Read the model definition and answer for the solid it produces. Units are mm, in the model's axes. Give positions to 0.01 mm unless a question says otherwise; leave off trailing zeros. Loops run counter-clockwise (first coordinate to the right, second up) from the corner with the lowest first, then second, coordinate; pieces in that order, holes last. Notation, with made-up numbers: (17, 61.25) -> (51, 61.25) arc R19 cw to (51, 69.25) -> close; hole circle Ø4 at (-24, 55). An arc over 180 degrees is marked (long way). One line per item, written item: value. Start each with the question number.
from build123d import *

# Parameters (mm, degrees)
SKETCH1_W      = 9.144
SKETCH1_H      = 4.572
EXTRUDE1_DEPTH = 3.048
SKETCH2_W      = 0.762
SKETCH2_H      = 0.762
EXTRUDE2_DEPTH = 7.62


with BuildPart() as part:
    # Sketch1 → Extrude1 (new body)
    with BuildSketch(Plane(origin=(0, 0, 0), x_dir=(1, 0, 0), z_dir=(0, 1, 0))):
        with Locations((4.572, 2.286)):
            Rectangle(SKETCH1_W, SKETCH1_H)
    extrude(amount=EXTRUDE1_DEPTH)

    # Sketch2 → Extrude2 (add)
    with BuildSketch(Plane(origin=(0, 3.048, 0), x_dir=(1, 0, 0), z_dir=(0, 1, 0))):
        with Locations((3.429, 3.429)):
            Rectangle(SKETCH2_W, SKETCH2_H)
        with Locations((1.143, 3.429)):
            Rectangle(SKETCH2_W, SKETCH2_H)
        with Locations((5.715, 3.429)):
            Rectangle(SKETCH2_W, SKETCH2_H)
        with Locations((8.001, 3.429)):
            Rectangle(SKETCH2_W, SKETCH2_H)
        with Locations((1.143, 1.143)):
            Rectangle(SKETCH2_W, SKETCH2_H)
        with Locations((3.429, 1.143)):
            Rectangle(SKETCH2_W, SKETCH2_H)
        with Locations((5.715, 1.143)):
            Rectangle(SKETCH2_W, SKETCH2_H)
        with Locations((8.001, 1.143)):
            Rectangle(SKETCH2_W, SKETCH2_H)
    extrude(amount=EXTRUDE2_DEPTH)


solid = part.part
Item 1: Section C-C, the plane x = 8.25 is taken. Determine the outline of the cut face in (y, z).
Item 2: Section A-A, the plane y = 5 is taken. State how many separate pieces and enclosed holes the cut face has, plus the area to 3 significant figures.
Item 3: Consider L1, parallel to X at y = 9.25, z = -3.4; L2, parallel to Z at x = 1.25, y = 5.5; L3, parallel to Y at x = 2, z = -3.15. Determine where each line is inside the solid, lowest interval first. Write a range as [from, to].
Item 4: Flat-ended cylindrical pins translate along their axes: pin 1 (0.8 mm diameter, centred on y = 7, z = -3.5, fed in from -X); pin 2 (0.6 mm diameter, centred on y = 7, z = -1, fed in from +X); pin 3 (1 mm diameter, centred on x = 8, y = 8, fed in from -Z). Find the tip coordinate at first contact, or state that the pin passes through.
Item 5: Determine the mould class of faces 1 (the flat face through (0, 2, -2)), 2 (the flat face through (9.144, 2, -2)), 3 (the flat face through (5, 3.048, -2)), 4 (the flat face through (5, 2, 0)) for opening direction X: pulls with the +X half, pulls with the -X half, needs draft (parallel to the pull), parting line crosses it, or undercut.
Item 6: Section D-D, the plane x = 6.5 is taken. Determine the outline of the cut face in (y, z), plus the area to 3 significant figures.
Item 7: Section B-B, the plane z = -1 is taken. Determine the outline of the cut face in (x, y), plus the area to 3 significant figures.
Computed values:
1. outline: (0, -4.57) -> (3.05, -4.57) -> (3.05, -3.81) -> (10.67, -3.81) -> (10.67, -3.05) -> (3.05, -3.05) -> (3.05, -1.52) -> (10.67, -1.52) -> (10.67, -0.76) -> (3.05, -0.76) -> (3.05, 0) -> (0, 0) -> close
2. separate pieces: 8
2. enclosed holes: 0
2. area: 4.65 mm²
3. L1: [0.76, 1.52], [3.05, 3.81], [5.33, 6.1], [7.62, 8.38]
3. L2: [-3.81, -3.05], [-1.52, -0.76]
3. L3: [0, 3.05]
4. pin 1: x = 0.76
4. pin 2: x = 8.38
4. pin 3: z = -3.81
5. face 1: pulls with the -X half
5. face 2: pulls with the +X half
5. face 3: undercut
5. face 4: needs draft
6. outline: (0, -4.57) -> (3.05, -4.57) -> (3.05, 0) -> (0, 0) -> close
6. area: 13.9 mm²
7. outline: (0, 0) -> (9.14, 0) -> (9.14, 3.05) -> (8.38, 3.05) -> (8.38, 10.67) -> (7.62, 10.67) -> (7.62, 3.05) -> (6.1, 3.05) -> (6.1, 10.67) -> (5.33, 10.67) -> (5.33, 3.05) -> (3.81, 3.05) -> (3.81, 10.67) -> (3.05, 10.67) -> (3.05, 3.05) -> (1.52, 3.05) -> (1.52, 10.67) -> (0.76, 10.67) -> (0.76, 3.05) -> (0, 3.05) -> close
7. area: 51.1 mm²
